The drawing under review shows one solid part. Ordinate dimensions are in mm from its lowest x, y, z. A direction names the side the tool comes from. Coordinates: 2 decimals unless noted, no trailing zeros. Loops run counter-clockwise (first coordinate to the right, second up) from the corner with the lowest first, then second, coordinate; pieces in that order, holes last.
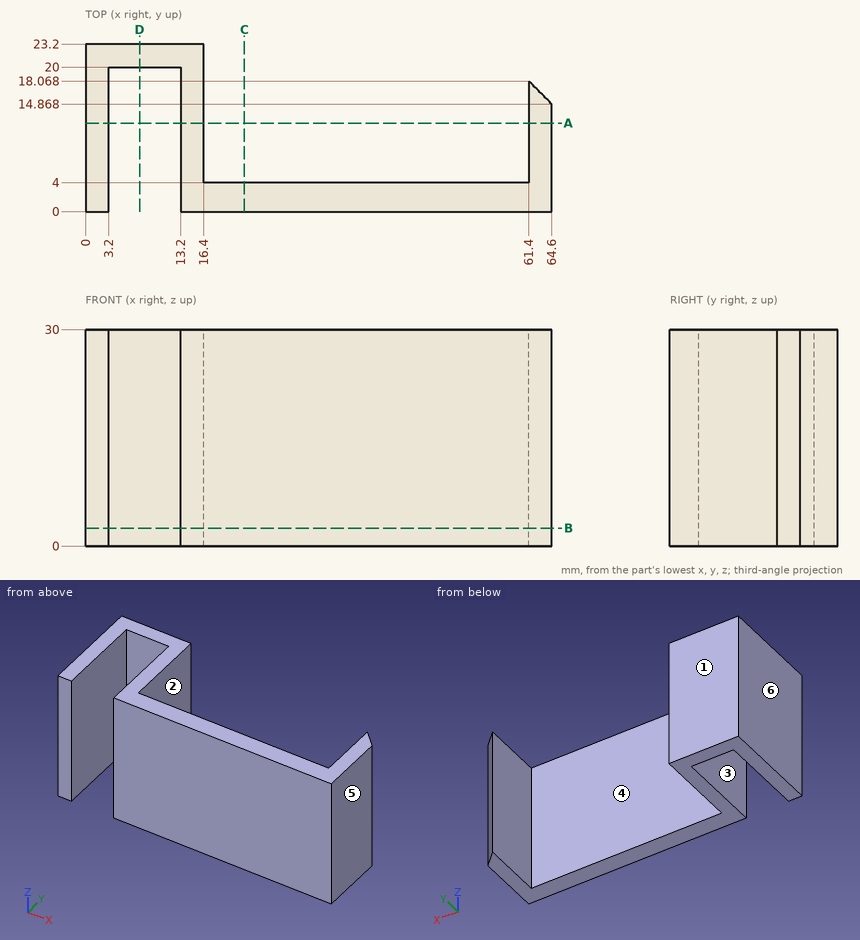
Q1. Take a section at D-D, the plane x = 7.5. Write out the cut boundary in (y, z), then the cut area to 3 significant figures.
Q2. Clearance check with flat-ended pins moving along their axes: pin 1 Ø10 at (x, z) = (47.5, 12) entering from +Y; pin 2 Ø3 at (x, z) = (9, 19) entering from -Y. State where each tip first meets the part, or that it passes through.
Q3. Take a section at B-B, the plane z = 2.5. Write out the cut boundary in (x, y), then the cut area to 3 significant figures.
Q4. Take a section at A-A, the plane y = 12.25. Write out the cut boundary in (x, z).
Q5. For line 1 (X direction, y = 13.25, z = 7); line 2 (X direction, y = 1.25, z = 25); line 3 (X direction, y = 15, z = 20), list the stretches that pass through material, from the lowest coordinate up.
Q6. Take a section at C-C, the plane x = 22. Write out the cut boundary in (y, z).
Q7. The part is to be moulded in two halves that separate along X. For the marked faces 4, 5 and 6, say which applies: pulls with the +X half, pulls with the -X half, needs draft (parallel to the pull), parting line crosses it, or undercut.
Q8. Machinability: for the marked faces 1, 2 and 3, which of the approach directions +Z, -Z, +X, -X, +Y, -Y give a long, thin tool a straight path to every point of the face, cutting with its end or side? Answer none if there is none.
Entries:
1. outline: (20, 0) - (23.2, 0) - (23.2, 30) - (20, 30) - close
1. area: 96.0 mm2
2. pin 1: stops at y = 4
2. pin 2: stops at y = 20
3. outline: (0, 0) - (3.2, 0) - (3.2, 20) - (13.2, 20) - (13.2, 0) - (64.6, 0) - (64.6, 14.87) - (61.4, 18.07) - (61.4, 4) - (16.4, 4) - (16.4, 23.2) - (0, 23.2) - close
3. area: 413 mm2
4. outline: (0, 0) - (3.2, 0) - (3.2, 30) - (0, 30) - close; (13.2, 0) - (16.4, 0) - (16.4, 30) - (13.2, 30) - close; (61.4, 0) - (64.6, 0) - (64.6, 30) - (61.4, 30) - close
5. line 1: x = 0 to 3.2, 13.2 to 16.4, 61.4 to 64.6
5. line 2: x = 0 to 3.2, 13.2 to 64.6
5. line 3: x = 0 to 3.2, 13.2 to 16.4, 61.4 to 64.47
6. outline: (0, 0) - (4, 0) - (4, 30) - (0, 30) - close
7. face 4: undercut
7. face 5: pulls with the +X half
7. face 6: pulls with the -X half
8. face 1: +Z, -Z, +X, -X, +Y
8. face 2: +Z, -Z, +Y
8. face 3: +Z, -Z, -Y
